```python
from build123d import *

# Parameters (mm, degrees)
F1_DEPTH = 3.175
F2_DEPTH = 3.175


with BuildPart() as f1:
    # F0 (on Top) → F1 (new body)
    with BuildSketch(Plane.XY):
        with BuildLine():
            ThreePointArc((1.5875, 12.7), (0, 11.1125), (-1.5875, 12.7))
            Line((-1.5875, 12.7), (-1.5875, -12.7))
            ThreePointArc((-1.5875, -12.7), (0, -11.1125), (1.5875, -12.7))
            Line((1.5875, -12.7), (1.5875, 12.7))
        make_face()
        with BuildLine():
            ThreePointArc((1.5875, -12.7), (0, -11.1125), (-1.5875, -12.7))
            Line((-1.5875, -12.7), (1.5875, -12.7))
        make_face()
        with BuildLine():
            Line((1.5875, -12.7), (-1.5875, -12.7))
            ThreePointArc((-1.5875, -12.7), (0, -14.2875), (1.5875, -12.7))
        make_face()
        with BuildLine():
            ThreePointArc((1.5875, 12.7), (0, 14.2875), (-1.5875, 12.7))
            Line((-1.5875, 12.7), (1.5875, 12.7))
        make_face()
        with BuildLine():
            Line((1.5875, 12.7), (-1.5875, 12.7))
            ThreePointArc((-1.5875, 12.7), (0, 11.1125), (1.5875, 12.7))
        make_face()
    extrude(amount=F1_DEPTH)

    # F0 (on Top) → F2 (join)
    with BuildSketch(Plane.XY):
        with BuildLine():
            Line((1.5875, -12.7), (-1.5875, -12.7))
            ThreePointArc((-1.5875, -12.7), (0, -14.2875), (1.5875, -12.7))
        make_face()
        with BuildLine():
            ThreePointArc((1.5875, -12.7), (0, -11.1125), (-1.5875, -12.7))
            Line((-1.5875, -12.7), (1.5875, -12.7))
        make_face()
    extrude(amount=-F2_DEPTH)


solid = f1.part
```
Could you check a few things on this model? Use its own coordinates, in mm. A direction names the side the tool comes from. Round coordinates to 2 decimals unless told otherwise and drop trailing zeros. Loops run counter-clockwise (first coordinate to the right, second up) from the corner with the lowest first, then second, coordinate; pieces in that order, holes last. Notation, with made-up numbers: (32, 9.25) - (91, 9.25) arc R30 cw to (91, 47.25) - close; hole circle Ø7 at (22.25, 50). An arc over 180 degrees is marked (long way). Answer as CSV lines item,"result".
1. I want a section at B-B on y = 1.75. List the corners of the cut face in (x, z) for me (1 decimal), then the cut area to 3 significant figures.
Filled in:
outline,"(-1.6, 0) - (1.6, 0) - (1.6, 3.2) - (-1.6, 3.2) - close"
area,"10.1 mm^2"
2. Please list where these lines run through material, in increasing order: line 1 along Z through (x, y) = (1.05, 9.25) (3 decimals); line 2 along Y through (x, z) = (0.1, -1.25); line 3 along Y through (x, z) = (-0.2, 0.5). Write a range as [from, to].
Filled in:
line 1,"z = [0, 3.175]"
line 2,"y = [-14.28, -11.12]"
line 3,"y = [-14.27, 14.27]"
3. I want a section at A-A on x = 0. List the corners of the cut face in (y, z) for me (1 decimal), then the cut area to 3 significant figures.
Filled in:
outline,"(-14.3, -3.2) - (-11.1, -3.2) - (-11.1, 0) - (14.3, 0) - (14.3, 3.2) - (-14.3, 3.2) - close"
area,"101 mm^2"
4. For pin 1 Ø1 at (x, y) = (-0.5, 3.5) entering from -Z, with a flat end and sliding along its axis, tell me the tip position at first contact or that it passes through.
Filled in:
pin 1,"stops at z = 0"
5. I want a section at C-C on z = 0.5. List the corners of the cut face in (x, y) for me (1 decimal).
Filled in:
outline,"(-1.6, -12.7) arc R1.6 ccw to (1.6, -12.7) - (1.6, 12.7) arc R1.6 ccw to (-1.6, 12.7) - close"
6. On a 3-axis mill with a long thin cutter (end or side, diameter ignored), from which of +Z, -Z, +X, -X, +Y, -Y can I reach the whole of each face in a straight line? I mean faces 1 (the face through (0.035, 14.287, 1.565)), 2 (the face through (-0.34, -14.25, -0.66)). Say none if no direction works.
Filled in:
face 1,"+Z, -Z, +Y"
face 2,"-Z"
7. I want a section at D-D on y = -11.5. List the corners of the cut face in (x, z) for me (1 decimal).
Filled in:
outline,"(-1.6, 0) - (-1, 0) - (-1, -3.2) - (1, -3.2) - (1, 0) - (1.6, 0) - (1.6, 3.2) - (-1.6, 3.2) - close"
